Geometry: final body of the model. Coordinates: model frame, mm. Face numbers are marked on the shaded views. Round coordinates to 2 decimals unless told otherwise and drop trailing zeros. Loops run counter-clockwise (first coordinate to the right, second up) from the corner with the lowest first, then second, coordinate; pieces in that order, holes last. Notation, with made-up numbers: (68, 46) -> (119, 46) arc R18 cw to (119, 66) -> close; hole circle Ø1 at (61, 62.25). An arc over 180 degrees is marked (long way). Answer in a Markdown table with one row per item.
```python
from build123d import *

# Parameters (mm, degrees)
SKETCH1_W                     = 110
SKETCH1_H                     = 5
BOSS_EXTRUDE1_DEPTH           = 70
M2_CLEARANCE_HOLE1_AT_2_COUNT = 2
M2_CLEARANCE_HOLE1_AT_2_PITCH = 50
SKETCH4_W                     = 2
SKETCH4_H                     = 5
CUT_EXTRUDE1_DEPTH            = 4.5


with BuildPart() as part:
    # Sketch1 → Boss-Extrude1 (new body)
    with BuildSketch(Plane.XY):
        with Locations((0, 16)):
            Rectangle(SKETCH1_W, SKETCH1_H)
    extrude(amount=BOSS_EXTRUDE1_DEPTH)

    # Sketch3 → M2 Clearance Hole1 (revolve, cut)
    with BuildSketch(Plane(origin=(-55, 16, 10), x_dir=(0, 0, 1), z_dir=(0, 1, 0))):
        Polygon((0, 0), (0, 9.721032743), (1.2, 9), (1.2, 0), align=None)
    m2_clearance_hole1 = revolve(axis=Axis((-61.35, 16, 10), (1, 0, 0)), mode=Mode.SUBTRACT)

    # M2 Clearance Hole1 at 2: M2 Clearance Hole1 ×2
    with Locations(*[(0, 0, i * M2_CLEARANCE_HOLE1_AT_2_PITCH) for i in range(1, M2_CLEARANCE_HOLE1_AT_2_COUNT)]):
        add(m2_clearance_hole1, mode=Mode.SUBTRACT)

    # Sketch4 → Cut-Extrude1 (cut)
    with BuildSketch(Plane(origin=(0, 18.5, 0), x_dir=(1, 0, 0), z_dir=(0, 1, 0))):
        with Locations((-45.4, -60)):
            Rectangle(SKETCH4_W, SKETCH4_H)
        with Locations((-45.4, -10)):
            Rectangle(SKETCH4_W, SKETCH4_H)
    cut_extrude1 = extrude(amount=-CUT_EXTRUDE1_DEPTH, mode=Mode.SUBTRACT)

    # Mirror1: M2 Clearance Hole1, Cut-Extrude1 across plane
    add(m2_clearance_hole1.mirror(Plane(origin=(0, 0, 0), x_dir=(0, 0, 1), z_dir=(1, 0, 0))), mode=Mode.SUBTRACT)
    add(cut_extrude1.mirror(Plane(origin=(0, 0, 0), x_dir=(0, 0, 1), z_dir=(1, 0, 0))), mode=Mode.SUBTRACT)

    # Mirror1 copy 1 sketch → Mirror1 copy 1 (revolve, cut)
    with BuildSketch(Plane(origin=(55, 16, 60), x_dir=(0, 0, 1), z_dir=(0, 1, 0))):
        Polygon((0, 0), (0, -9.721032743), (1.2, -9), (1.2, 0), align=None)
    revolve(axis=Axis((61.35, 16, 60), (1, 0, 0)), mode=Mode.SUBTRACT)


solid = part.part
```
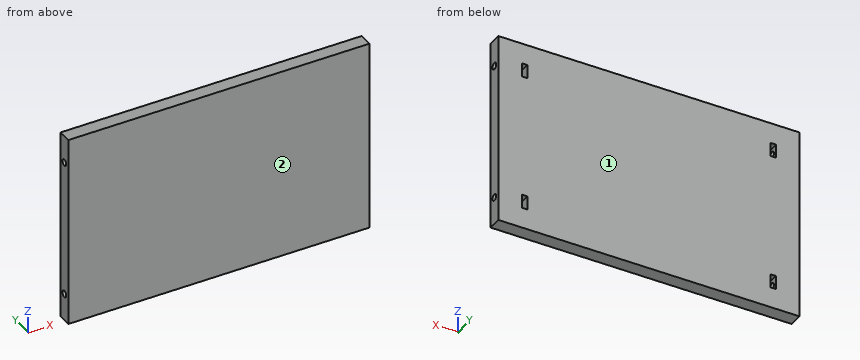
Item 1: Cut plane A-A (z = 10). Output: boundary loops of the cut face in (x, y).
Answer:
| item | result |
|---|---|
| outline | (-55, 13.5) -> (55, 13.5) -> (55, 14.8) -> (46.4, 14.8) -> (46.4, 14) -> (44.4, 14) -> (44.4, 18.5) -> (-44.4, 18.5) -> (-44.4, 14) -> (-46.4, 14) -> (-46.4, 14.8) -> (-55, 14.8) -> close; (-55, 17.2) -> (-46.4, 17.2) -> (-46.4, 18.5) -> (-55, 18.5) -> close; (46.4, 17.2) -> (55, 17.2) -> (55, 18.5) -> (46.4, 18.5) -> close |
Item 2: Draft query along Y for the marked faces 1 and 2. Return one class per face: pulls with the +Y half, pulls with the -Y half, needs draft (parallel to the pull), parting line crosses it, or undercut.
Answer:
| item | result |
|---|---|
| face 1 | pulls with the +Y half |
| face 2 | pulls with the -Y half |
Item 3: Line query: probe 1 along X at (y, z) = (15.9, 12); probe 2 along Z at (x, y) = (51.75, 16); probe 3 along Y at (x, z) = (-52, 60). Output: solid intervals per line, ascending. Write a range as [from, to].
Answer:
| item | result |
|---|---|
| probe 1 | x = [-55, -46.4], [-44.4, 44.4], [46.4, 55] |
| probe 2 | z = [0, 8.8], [11.2, 58.8], [61.2, 70] |
| probe 3 | y = [13.5, 14.8], [17.2, 18.5] |
Item 4: Pin query (flat end, axial travel): pin 1 Ø1.9 at (y, z) = (16, 60) entering from +X; pin 2 Ø1.6 at (x, z) = (45.5, 9) entering from +Y; pin 3 Ø2 at (y, z) = (16, 10) entering from -X. Return the tip coordinate at first contact, or that it passes through.
Answer:
| item | result |
|---|---|
| pin 1 | stops at x = 44.4 |
| pin 2 | stops at y = 14 |
| pin 3 | stops at x = -44.4 |
